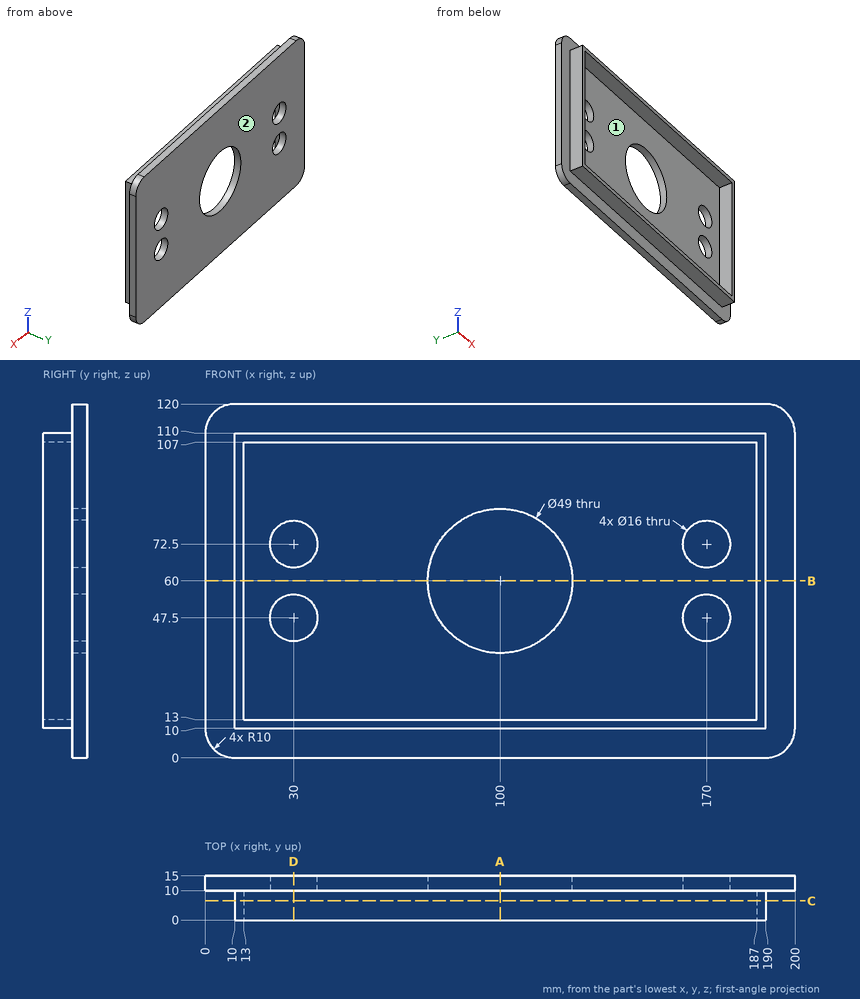
Part print with two shaded views. Sizes in mm from the minimum x, y, z corner. Coordinates: 2 decimals unless noted, no trailing zeros. Write each loop counter-clockwise with the first axis right and the second up, starting at its lowest first coordinate (ties: lowest second). Pieces come first, ordered by that corner, then holes.
(1) Mould opens along Z. For the marked faces 1 and 2 say: pulls with the +Z half, pulls with the -Z half, needs draft (parallel to the pull), parting line crosses it, or undercut.
(2) Pin check, flat tips, straight feed: pin 1 Ø1.5 at (y, z) = (8.5, 15.5) entering from +X; pin 2 Ø5 at (x, y) = (81.5, 5.5) entering from -Z; pin 3 Ø4 at (y, z) = (7, 39.5) entering from -X. Stop position of each tip, or through.
(3) Cut at A-A on x = 100. List the corners of the cut face in (y, z), and give its area (3 significant figures).
(4) Cut at B-B on z = 60. List the corners of the cut face in (x, y).
(5) Cut at C-C on y = 6.5. List the corners of the cut face in (x, z), and give its area (3 significant figures).
(6) Cut at D-D on x = 30. List the corners of the cut face in (y, z).
(7) Drill centre lines: line 1 (Z direction, x = 170, y = 11.3); line 2 (X direction, y = 7.5, z = 77); line 3 (Z direction, x = 74.5, y = 5.25). Where is each one in solid material? Low to high.
Working result:
1. face 1: undercut
1. face 2: needs draft
2. pin 1: stops at x = 190
2. pin 2: stops at z = 10
2. pin 3: stops at x = 10
3. outline: (0, 10) - (10, 10) - (10, 0) - (15, 0) - (15, 35.5) - (10, 35.5) - (10, 13) - (0, 13) - close; (0, 107) - (10, 107) - (10, 84.5) - (15, 84.5) - (15, 120) - (10, 120) - (10, 110) - (0, 110) - close
3. area: 415 mm2
4. outline: (0, 10) - (10, 10) - (10, 0) - (13, 0) - (13, 10) - (75.5, 10) - (75.5, 15) - (0, 15) - close; (124.5, 10) - (187, 10) - (187, 0) - (190, 0) - (190, 10) - (200, 10) - (200, 15) - (124.5, 15) - close
5. outline: (10, 10) - (190, 10) - (190, 110) - (10, 110) - close; hole (13, 13) - (187, 13) - (187, 107) - (13, 107) - close
5. area: 1,640 mm2
6. outline: (0, 10) - (10, 10) - (10, 0) - (15, 0) - (15, 39.5) - (10, 39.5) - (10, 13) - (0, 13) - close; (0, 107) - (10, 107) - (10, 80.5) - (15, 80.5) - (15, 120) - (10, 120) - (10, 110) - (0, 110) - close; (10, 55.5) - (15, 55.5) - (15, 64.5) - (10, 64.5) - close
7. line 1: z = 0 to 39.5, 55.5 to 64.5, 80.5 to 120
7. line 2: x = 10 to 13, 187 to 190
7. line 3: z = 10 to 13, 107 to 110
